from build123d import *

# Parameters (mm, degrees)
F0_W     = 10.518072
F0_H     = 0.8
F0_H_2   = 1
F1_DEPTH = 1.3
F2_DEPTH = 4.75


with BuildPart() as f1:
    # F0 (on Top) → F1 (new body)
    with BuildSketch(Plane.XY):
        with Locations((0, 1.8)):
            Rectangle(F0_W, F0_H)
        with Locations((0, 0.9)):
            Rectangle(F0_W, F0_H_2)
        Rectangle(F0_W, F0_H)
        with Locations((0, -0.9)):
            Rectangle(F0_W, F0_H_2)
        with Locations((0, -1.8)):
            Rectangle(F0_W, F0_H)
        with Locations((0, -2.7)):
            Rectangle(F0_W, F0_H_2)
        with Locations((0, -3.6)):
            Rectangle(F0_W, F0_H)
    extrude(amount=F1_DEPTH)

    # F0 (on Top) → F2 (join)
    with BuildSketch(Plane.XY):
        with Locations((0, 1.8)):
            Rectangle(F0_W, F0_H)
        Rectangle(F0_W, F0_H)
        with Locations((0, -1.8)):
            Rectangle(F0_W, F0_H)
        with Locations((0, -3.6)):
            Rectangle(F0_W, F0_H)
    extrude(amount=F2_DEPTH)


solid = f1.part
Geometry: final body of the model. Coordinates: model frame, mm. A direction names the side the tool comes from. Coordinates: 2 decimals unless noted, no trailing zeros. Loops run counter-clockwise (first coordinate to the right, second up) from the corner with the lowest first, then second, coordinate; pieces in that order, holes last. Notation, with made-up numbers: M -36,8.5 L 10,8.5 A27 ccw 10,33.5 Z; hole C -35.5,30 d4. An arc over 180 degrees is marked long. One line per item, written item: value. Start each with the question number.
1) Cut plane B-B (x = -3.5). Return loops of the section in (y, z), then the cut area to 3 significant figures.
2) Reachability of faces 1 (the flat face through (0, -2, 4.75)), 2 (the flat face through (0, -1, 1.3)) from +Z, -Z, +X, -X, +Y, -Y: full face, straight path, thin tool, end or side. Return the list, or none.
3) Draft query along Y for faces 3 (the flat face through (0, -4, 2)), 4 (the flat face through (0, -2.2, 3)), 5 (the flat face through (0, 2.2, 2)), 6 (the flat face through (5.259, -1, 1)). Return one class per face: released by +Y, released by -Y, zero draft, split by the parting line, or undercut.
4) Cut plane C-C (y = 1). Return loops of the section in (x, z), then the cut area to 3 significant figures.
5) Cut plane A-A (z = 3). Return loops of the section in (x, y), then the cut area to 3 significant figures.
6) Material intervals for L1, parallel to Y at x = -3.5, z = 4.35; L2, parallel to Z at x = -3, y = -1, sorted ascending. Write a range as from..to.
7) Pin query (flat end, axial travel): P1, Ø0.5, axis at x = 1.5, y = 1, coming from the +Z side. Return the tip coordinate at first contact, or that it passes through.
Evaluation:
1. outline: M -4,0 L 2.2,0 L 2.2,4.75 L 1.4,4.75 L 1.4,1.3 L 0.4,1.3 L 0.4,4.75 L -0.4,4.75 L -0.4,1.3 L -1.4,1.3 L -1.4,4.75 L -2.2,4.75 L -2.2,1.3 L -3.2,1.3 L -3.2,4.75 L -4,4.75 Z
1. area: 19.1 mm^2
2. face 1: +Z, +X, -X, +Y, -Y
2. face 2: +Z, +X, -X
3. face 3: released by -Y
3. face 4: undercut
3. face 5: released by +Y
3. face 6: zero draft
4. outline: M -5.26,0 L 5.26,0 L 5.26,1.3 L -5.26,1.3 Z
4. area: 13.7 mm^2
5. outline: M -5.26,-4 L 5.26,-4 L 5.26,-3.2 L -5.26,-3.2 Z; M -5.26,-2.2 L 5.26,-2.2 L 5.26,-1.4 L -5.26,-1.4 Z; M -5.26,-0.4 L 5.26,-0.4 L 5.26,0.4 L -5.26,0.4 Z; M -5.26,1.4 L 5.26,1.4 L 5.26,2.2 L -5.26,2.2 Z
5. area: 33.7 mm^2
6. L1: -4..-3.2, -2.2..-1.4, -0.4..0.4, 1.4..2.2
6. L2: 0..1.3
7. P1: z = 1.3
